Check sheet for the drawn part. Datum: minimum x, y, z corner. Units: mm. Round coordinates to 2 decimals unless told otherwise and drop trailing zeros. Order: outer loops, then holes, each group sorted by start corner. A loop starts at its lowest first (then second) coordinate and runs counter-clockwise, first axis right, second up.
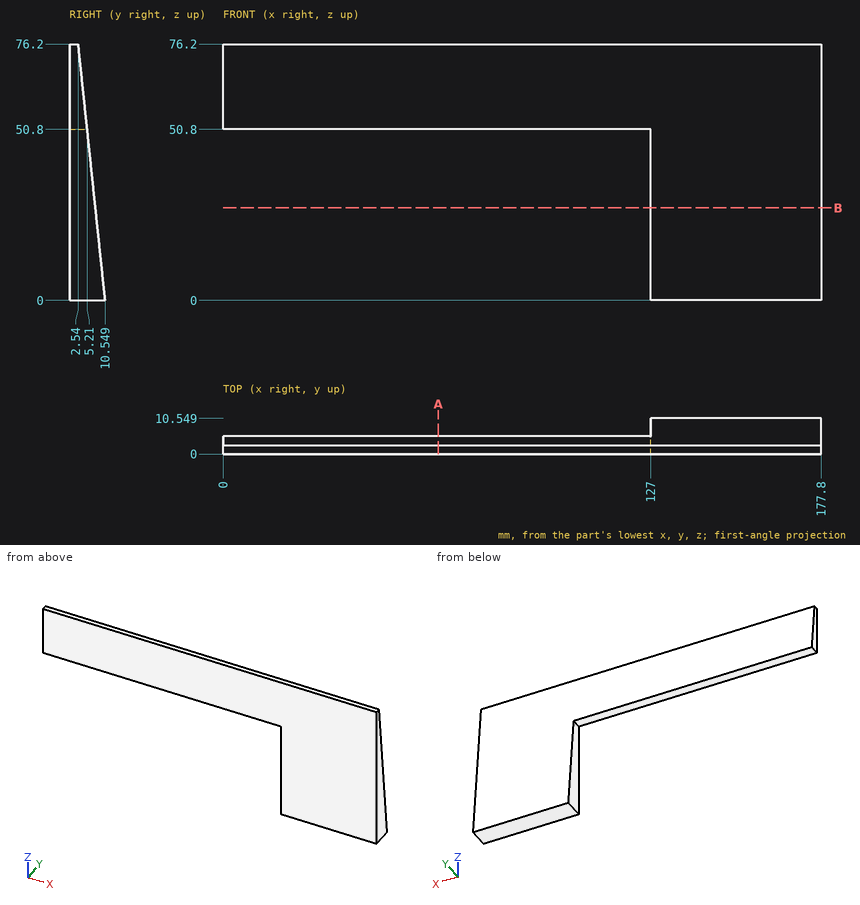
(1) Sectioned sample at A-A, the plane x = 64. Record the cut outline in (y, z).
Returned:
outline: (0, 50.8) - (5.21, 50.8) - (2.54, 76.2) - (0, 76.2) - close
(2) Material ranges on line 1 (X direction, y = 4.25, z = 43.5); line 2 (Y direction, x = 64, z = 53); line 3 (Y direction, x = 137, z = 19.5), recorded low to high.
Returned:
line 1: x = 127 to 177.8
line 2: y = 0 to 4.98
line 3: y = 0 to 8.5
(3) Depth check by flat-ended pin: P1, Ø3, axis at x = 107, y = 8.5, coming from the -Z side; P2, Ø3, axis at y = 7.5, z = 17, coming from the -X side; P3, Ø1.6, axis at x = 48.5, y = 2, coming from the -Z side. Enter the tip coordinate at first touch or a pass-through.
Returned:
P1: passes through
P2: stops at x = 127
P3: stops at z = 50.8
(4) Sectioned sample at B-B, the plane z = 27.5. Record the cut outline in (x, y).
Returned:
outline: (127, 0) - (177.8, 0) - (177.8, 7.66) - (127, 7.66) - close
